The drawing under review shows one solid part. Ordinate dimensions are in mm from its lowest x, y, z. A direction names the side the tool comes from. Coordinates: 2 decimals unless noted, no trailing zeros. Write each loop counter-clockwise with the first axis right and the second up, starting at its lowest first coordinate (ties: lowest second). Pieces come first, ordered by that corner, then holes.
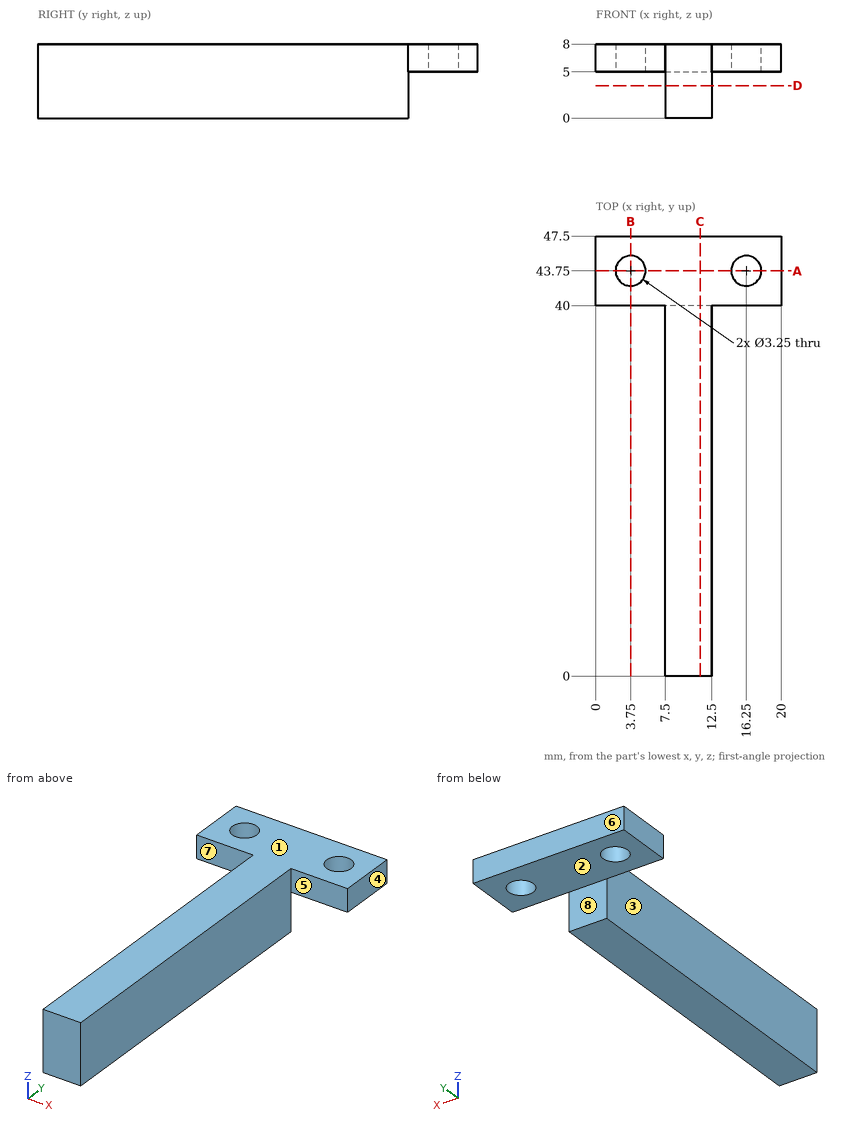
1) For L1, parallel to Y at x = 16.25, z = 6.2 (3 decimals); L2, parallel to Y at x = 19, z = 5.25; L3, parallel to X at y = 4, z = 2, list the stretches that pass through material, from the lowest coordinate up.
2) Tool access review of the marked faces 4, 5, 6, 7 and 8: name each direction out of +Z, -Z, +X, -X, +Y, -Y from which nothing blocks a thin tool from reaching the whole face with its end or side.
3) Clearance check with flat-ended pins moving along their axes: P1, Ø1, axis at y = 32.5, z = 3.5, coming from the -X side; P2, Ø2, axis at x = 11, y = 45.5, coming from the -Z side; P3, Ø2.5, axis at x = 9.5, z = 2.5, coming from the +Y side. State where each tip first meets the part, or that it passes through.
4) Consider section B-B (x = 3.75). Give the boundary of the cut face in (y, z) (3 decimals), then the cut area to 4 significant figures.
5) Consider section A-A (y = 43.75). Give the boundary of the cut face in (x, z) (3 decimals), then the cut area to 3 significant figures.
6) The part is to be moulded in two halves that separate along Z. For the marked faces 1, 2 and 3, say which applies: pulls with the +Z half, pulls with the -Z half, needs draft (parallel to the pull), parting line crosses it, or undercut.
7) Consider section D-D (z = 3.5). Give the boundary of the cut face in (x, y), then the cut area to 3 significant figures.
8) Consider section C-C (x = 11.25). Give the boundary of the cut face in (y, z), then the cut area to 4 significant figures.
Results:
1. L1: y = 40 to 42.125, 45.375 to 47.5
1. L2: y = 40 to 47.5
1. L3: x = 7.5 to 12.5
2. face 4: +Z, -Z, +X, +Y, -Y
2. face 5: +Z, -Z, +X, -Y
2. face 6: +Z, -Z, +X, -X, +Y
2. face 7: +Z, -Z, -X, -Y
2. face 8: -Z, +X, -X, +Y
3. P1: stops at x = 7.5
3. P2: stops at z = 5
3. P3: stops at y = 40
4. outline: (40, 5) - (42.125, 5) - (42.125, 8) - (40, 8) - close; (45.375, 5) - (47.5, 5) - (47.5, 8) - (45.375, 8) - close
4. area: 12.75 mm2
5. outline: (0, 5) - (2.125, 5) - (2.125, 8) - (0, 8) - close; (5.375, 5) - (14.625, 5) - (14.625, 8) - (5.375, 8) - close; (17.875, 5) - (20, 5) - (20, 8) - (17.875, 8) - close
5. area: 40.5 mm2
6. face 1: pulls with the +Z half
6. face 2: pulls with the -Z half
6. face 3: needs draft
7. outline: (7.5, 0) - (12.5, 0) - (12.5, 40) - (7.5, 40) - close
7. area: 200 mm2
8. outline: (0, 0) - (40, 0) - (40, 5) - (47.5, 5) - (47.5, 8) - (0, 8) - close
8. area: 342.5 mm2
